Here's how the part is built. I have some questions about the finished solid (model axes, mm). Face numbers are marked on the shaded views. Round coordinates to 2 decimals unless told otherwise and drop trailing zeros. Order: outer loops, then holes, each group sorted by start corner. A loop starts at its lowest first (then second) coordinate and runs counter-clockwise, first axis right, second up. Notation, with made-up numbers: (37, 85.5) - (92, 85.5) arc R22 cw to (92, 124.5) - close; hole circle Ø9 at (52.5, 10.25). An arc over 180 degrees is marked (long way). One line per item, written item: value.
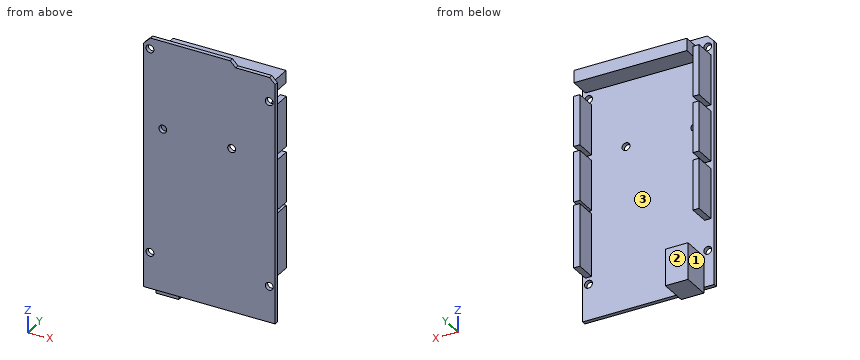
Autodesk Inventor part; units mm, degrees
ref_plane "YZ Plane" through (0, 0, 0) normal (1, 0, 0) x (0, 1, 0)
ref_plane "XZ Plane" through (0, 0, 0) normal (0, 1, 0) x (-1, 0, 0)
ref_plane "XY Plane" through (0, 0, 0) normal (0, 0, 1) x (1, 0, 0)
sketch "Sketch1" plane through (0, 0, 0) normal (0, 1, 0) x (-1, 0, 0)
  line L0 (-26.605, -50.8) -> (26.605, -50.8)
  line L1 (26.605, -50.8) -> (26.605, 48.05)
  line L2 (23.855, 50.8) -> (-8.395, 50.8)
  line L3 (-26.605, 46.3) -> (-26.605, -50.8)
  line L4 (26.605, 48.05) -> (23.855, 50.8)
  line L5 (-8.395, 50.8) -> (-10.645, 48.55)
  line L6 (-10.645, 48.55) -> (-24.355, 48.55)
  line L7 (-24.355, 48.55) -> (-26.605, 46.3)
  circle A0 centre (24.065, -36.2) radius 1.59
  circle A1 centre (18.855, 15.3) radius 1.59
  circle A2 centre (-24.195, 38.73) radius 1.59
  circle A3 centre (24.065, 46.35) radius 1.59
  circle A4 centre (-8.995, 15.3) radius 1.59
  circle A5 centre (-24.195, -36.2) radius 1.59
  line L8 (24.065, -36.2) -> (24.065, 46.35) construction
  line L9 (24.065, -36.2) -> (-24.195, -36.2) construction
  line L10 (-24.195, -36.2) -> (-24.195, 38.73) construction
  line L11 (18.855, 15.3) -> (-8.995, 15.3) construction
  point P0 (0, 0)
  dimension "d4" = 2.25
  dimension "d5" = 45
  dimension "d6" = 2.25
  dimension "d7" = 45
  dimension "d8" = 2.75
  dimension "d9" = 35
  dimension "d10" = 53.21
  dimension "d11" = 101.6
  dimension "d12" = 50.8
  dimension "d13" = 26.605
  dimension "d14" = 2.54
  dimension "d15" = 7.75
  dimension "d16" = 82.55
  dimension "d17" = 74.93
  dimension "d18" = 48.26
  dimension "d19" = 66.1
  dimension "d20" = 3.18
  dimension "d21" = 27.85
  dimension "d22" = 14.6
extrude "Extrusion1" add sketch "Sketch1" against normal blind 1.65
sketch "Sketch2" plane through (0, 0, 0) normal (0, 1, 0) x (1, 0, 0)
  circle A0 centre (24.195, 36.2) radius 1.59
  circle A1 centre (8.995, -15.3) radius 1.59
  circle A2 centre (-24.065, -46.35) radius 1.59
  circle A3 centre (24.195, -38.73) radius 1.59
  circle A4 centre (-18.855, -15.3) radius 1.59
  circle A5 centre (-24.065, 36.2) radius 1.59
  line L0 (26.605, 50.8) -> (-26.605, 50.8)
  line L1 (-26.605, 50.8) -> (-26.605, -48.05)
  line L2 (-26.605, -48.05) -> (-23.855, -50.8)
  line L3 (-23.855, -50.8) -> (8.395, -50.8)
  line L4 (8.395, -50.8) -> (10.645, -48.55)
  line L5 (10.645, -48.55) -> (24.355, -48.55)
  line L6 (24.355, -48.55) -> (26.605, -46.3)
  line L7 (26.605, -46.3) -> (26.605, 50.8)
  circle A6 centre (24.195, 36.2) radius 1.59
  line L8 (24.195, 36.2) -> (24.195, -38.73) construction
  line L9 (25.445, 7.9669) -> (22.945, 7.9669)
  line L10 (22.945, 7.9669) -> (22.945, 33.3669)
  line L11 (22.945, 33.3669) -> (25.445, 33.3669)
  line L12 (25.445, 33.3669) -> (25.445, 7.9669)
  line L13 (25.445, 7.9669) -> (22.945, 33.3669) construction
  line L14 (22.945, 7.9669) -> (25.445, 33.3669) construction
  line L15 (22.945, -13.6564) -> (25.445, -13.6564)
  line L16 (25.445, -13.6564) -> (25.445, 6.6636)
  line L17 (25.445, 6.6636) -> (22.945, 6.6636)
  line L18 (22.945, 6.6636) -> (22.945, -13.6564)
  line L19 (22.945, -13.6564) -> (25.445, 6.6636) construction
  line L20 (25.445, -13.6564) -> (22.945, 6.6636) construction
  line L21 (22.945, -36.2234) -> (25.445, -36.2234)
  line L22 (25.445, -36.2234) -> (25.445, -15.9034)
  line L23 (25.445, -15.9034) -> (22.945, -15.9034)
  line L24 (22.945, -15.9034) -> (22.945, -36.2234)
  line L25 (22.945, -36.2234) -> (25.445, -15.9034) construction
  line L26 (25.445, -36.2234) -> (22.945, -15.9034) construction
  line L27 (-20.3658, -46.7367) -> (25.3542, -46.7367)
  line L28 (25.3542, -46.7367) -> (25.3542, -41.7367)
  line L29 (25.3542, -41.7367) -> (-20.3658, -41.7367)
  line L30 (-20.3658, -41.7367) -> (-20.3658, -46.7367)
  line L31 (-20.3658, -46.7367) -> (25.3542, -41.7367) construction
  line L32 (25.3542, -46.7367) -> (-20.3658, -41.7367) construction
  circle A7 centre (-24.065, 36.2) radius 1.59
  line L33 (-24.065, 36.2) -> (-24.065, -46.35) construction
  line L34 (-25.315, 3.37) -> (-22.815, 3.37)
  line L35 (-22.815, 3.37) -> (-22.815, 23.69)
  line L36 (-22.815, 23.69) -> (-25.315, 23.69)
  line L37 (-25.315, 23.69) -> (-25.315, 3.37)
  line L38 (-25.315, 3.37) -> (-22.815, 23.69) construction
  line L39 (-22.815, 3.37) -> (-25.315, 23.69) construction
  line L40 (-25.315, -19.9342) -> (-22.815, -19.9342)
  line L41 (-22.815, -19.9342) -> (-22.815, 0.3858)
  line L42 (-22.815, 0.3858) -> (-25.315, 0.3858)
  line L43 (-25.315, 0.3858) -> (-25.315, -19.9342)
  line L44 (-25.315, -19.9342) -> (-22.815, 0.3858) construction
  line L45 (-22.815, -19.9342) -> (-25.315, 0.3858) construction
  line L46 (-25.315, -42.7584) -> (-22.815, -42.7584)
  line L47 (-22.815, -42.7584) -> (-22.815, -22.4384)
  line L48 (-22.815, -22.4384) -> (-25.315, -22.4384)
  line L49 (-25.315, -22.4384) -> (-25.315, -42.7584)
  line L50 (-25.315, -42.7584) -> (-22.815, -22.4384) construction
  line L51 (-22.815, -42.7584) -> (-25.315, -22.4384) construction
  point P0 (0, 0)
  point P1 (24.195, 20.6669)
  point P2 (24.195, -3.4964)
  point P3 (24.195, -26.0634)
  point P4 (2.4942, -44.2367)
  point P5 (-24.065, 13.53)
  point P6 (-24.065, -9.7742)
  point P7 (-24.065, -32.5984)
  dimension "d23" = 25.4
  dimension "d24" = 20.32
  dimension "d25" = 2.5
  dimension "d26" = 20.32
  dimension "d27" = 5
  dimension "d28" = 45.72
  dimension "d29" = 20.32
  dimension "d30" = 20.32
  dimension "d31" = 20.32
extrude "Extrusion2" add sketch "Sketch2" along normal blind 8.3 contours L9 L10 L11 L12 | L18 L17 L16 L15 | L24 L23 L22 L21 | L30 L29 L28 L27 | L37 L36 L35 L34 | L43 L42 L41 L40 | L49 L48 L47 L46
sketch "Sketch3" plane through (0, 0, 0) normal (0, 1, 0) x (1, 0, 0)
  line L0 (22.945, 7.9669) -> (22.945, 33.3669)
  line L1 (22.945, 33.3669) -> (25.445, 33.3669)
  line L2 (25.445, 33.3669) -> (25.445, 7.9669)
  line L3 (25.445, 7.9669) -> (22.945, 7.9669)
  line L4 (-25.315, -19.9342) -> (-25.315, 0.3858)
  line L5 (-25.315, 0.3858) -> (-22.815, 0.3858)
  line L6 (-22.815, 0.3858) -> (-22.815, -19.9342)
  line L7 (-22.815, -19.9342) -> (-25.315, -19.9342)
  line L8 (22.945, -36.2234) -> (22.945, -15.9034)
  line L9 (22.945, -15.9034) -> (25.445, -15.9034)
  line L10 (25.445, -15.9034) -> (25.445, -36.2234)
  line L11 (25.445, -36.2234) -> (22.945, -36.2234)
  line L12 (22.945, -13.6564) -> (22.945, 6.6636)
  line L13 (22.945, 6.6636) -> (25.445, 6.6636)
  line L14 (25.445, 6.6636) -> (25.445, -13.6564)
  line L15 (25.445, -13.6564) -> (22.945, -13.6564)
  line L16 (-25.315, 3.37) -> (-25.315, 23.69)
  line L17 (-25.315, 23.69) -> (-22.815, 23.69)
  line L18 (-22.815, 23.69) -> (-22.815, 3.37)
  line L19 (-22.815, 3.37) -> (-25.315, 3.37)
  line L20 (-25.315, -42.7584) -> (-25.315, -22.4384)
  line L21 (-25.315, -22.4384) -> (-22.815, -22.4384)
  line L22 (-22.815, -22.4384) -> (-22.815, -42.7584)
  line L23 (-22.815, -42.7584) -> (-25.315, -42.7584)
  line L24 (-20.3658, -46.7367) -> (-20.3658, -41.7367)
  line L25 (-20.3658, -41.7367) -> (25.3542, -41.7367)
  line L26 (25.3542, -41.7367) -> (25.3542, -46.7367)
  line L27 (25.3542, -46.7367) -> (-20.3658, -46.7367)
  circle A0 centre (24.195, 36.2) radius 1.59
  circle A1 centre (8.995, -15.3) radius 1.59
  circle A2 centre (-24.065, -46.35) radius 1.59
  circle A3 centre (24.195, -38.73) radius 1.59
  circle A4 centre (-18.855, -15.3) radius 1.59
  circle A5 centre (-24.065, 36.2) radius 1.59
  line L28 (26.605, 50.8) -> (-26.605, 50.8)
  line L29 (-26.605, 50.8) -> (-26.605, -48.05)
  line L30 (-26.605, -48.05) -> (-23.855, -50.8)
  line L31 (-23.855, -50.8) -> (8.395, -50.8)
  line L32 (8.395, -50.8) -> (10.645, -48.55)
  line L33 (10.645, -48.55) -> (24.355, -48.55)
  line L34 (24.355, -48.55) -> (26.605, -46.3)
  line L35 (26.605, -46.3) -> (26.605, 50.8)
  line L36 (-13.335, 53.1213) -> (-22.475, 53.1213)
  line L37 (-22.475, 53.1213) -> (-22.475, 38.2805)
  line L38 (-22.475, 38.2805) -> (-13.335, 38.2805)
  line L39 (-13.335, 38.2805) -> (-13.335, 53.1213)
  point P0 (0, 0)
  dimension "d34" = 9.14
extrude "Extrusion3" add sketch "Sketch3" along normal blind 11.18 contours L39 L38 L37 L28 | L28 L37 L36 L39
properties part number "Arduino Due"
Q1. If we section it at B-B, the plane y = 1.5: Give the number of separate pieces and of enclosed holes in the cut face, then the cut area to 3 significant figures.
Results list:
separate pieces: 8
enclosed holes: 0
area: 682 mm²
Q2. If we section it at D-D, the plane x = 12: Please give me the cut outline in (y, z), then the cut area to 3 significant figures.
Results list:
outline: (-1.65, -50.8) - (0, -50.8) - (0, 41.74) - (8.3, 41.74) - (8.3, 46.74) - (0, 46.74) - (0, 48.55) - (-1.65, 48.55) - close
area: 205 mm²
Q3. If I drill on line 1 along Z through (x, y) = (24.5, 6.5); line 2 along Z through (x, y) = (-23, -1); line 3 along X through (y, z) = (5.75, -19.5) (3 decimals), over which ranges is the centre line in solid material (lowest first)?
Results list:
line 1: -33.37 to -7.97, -6.66 to 13.66, 15.9 to 36.22, 41.74 to 46.74
line 2: -50.8 to -37.38, -35.02 to 45.17, 47.53 to 50.8
line 3: -25.315 to -22.815, 22.945 to 25.445
Q4. Will these pins go through, and if not, where does the flat tip stop? pin 1 (3 mm diameter, centred on x = 16, z = 27, fed in from +Y); pin 2 (3 mm diameter, centred on x = 24.5, y = 3, fed in from +Z); pin 3 (1.8 mm diameter, centred on x = 1, y = -0.5, fed in from -Z); pin 4 (1.9 mm diameter, centred on x = 8.995, z = 15.3, fed in from +Y).
Results list:
pin 1: y = 0
pin 2: z = 46.74
pin 3: z = -50.8
pin 4: through
Q5. If we section it at C-C, the plane z = -36.2: Please give me the cut outline in (x, y) (3 decimals), then the cut area to 3 significant figures.
Results list:
outline: (-26.605, -1.65) - (-25.655, -1.65) - (-25.655, 0) - (-26.605, 0) - close; (-22.475, -1.65) - (22.605, -1.65) - (22.605, 0) - (-22.475, 0) - close; (25.785, -1.65) - (26.605, -1.65) - (26.605, 0) - (25.785, 0) - close
area: 77.3 mm²
Q6. We'd pull the mould along X, two halves only. Please class the marked faces 1, 2 and 3: released by +X, released by -X, zero draft, split by the parting line, or undercut.
Results list:
face 1: released by -X
face 2: zero draft
face 3: undercut
Q7. If we section it at A-A, the plane z = 38.73: Please give me the cut outline in (x, y) (3 decimals).
Results list:
outline: (-26.605, -1.65) - (22.605, -1.65) - (22.605, 0) - (-22.815, 0) - (-22.815, 8.3) - (-25.315, 8.3) - (-25.315, 0) - (-26.605, 0) - close; (25.785, -1.65) - (26.605, -1.65) - (26.605, 0) - (25.785, 0) - close
